Verification items for the finished model (mm, model axes). A direction names the side the tool comes from. Give positions to 0.01 mm unless a question says otherwise; leave off trailing zeros. Write each loop counter-clockwise with the first axis right and the second up, starting at its lowest first coordinate (ties: lowest second). Pieces come first, ordered by that corner, then holes. Notation, with made-up numbers: (31.25, 45) - (66.25, 45) arc R33 ccw to (66.25, 74) - close; hole circle Ø7 at (15, 8). An arc over 180 degrees is marked (long way). Answer as a JSON object with one key per item and string values. Group by question number.
Item 1: Go/stop test with a flat-tipped pin: pin 1 (9.5 mm diameter, centred on x = 59.82, y = 20.1, fed in from -Z). Record where the tip stops, or that it passes through.
Item 2: Draft check along Y on faces 3 (the face through (35, 39.933, 5)), 4 (the face through (36, 24.503, 5)), 5 (the face through (9.02, 14.24, 4.93)), 6 (the face through (0, 20, 5)). Enter one of: +Y half, -Y half, draft (parallel to the pull), parting line (faces both ways), or undercut.
Item 3: Sectioned sample at B-B, the plane y = 17.5. Record the boundary of the cut face in (x, z).
Item 4: Tool access check on faces 1 (the face through (36, 15.695, 5)), 2 (the face through (68.865, 22.222, 8.521)). Record the directions out of +Z, -Z, +X, -X, +Y, -Y that give a thin tool (end or side, any length) a straight path to the whole face; none if there is none.
Item 5: Sectioned sample at D-D, the plane x = 5. Record the boundary of the cut face in (y, z).
Item 6: Sectioned sample at C-C, the plane z = 2. Record the boundary of the cut face in (x, y), and give its area (3 significant figures).
Item 7: Sectioned sample at A-A, the plane x = 34. Record the boundary of the cut face in (y, z), and give its area (3 significant figures).
Item 8: Scan lines: line 1 along Y through (x, z) = (39, 1.5); line 2 along X through (y, z) = (22.5, 9.5); line 3 along X through (y, z) = (17.5, 1.5). Record each from-to range of solid material in increasing order. Write a range as [from, to].
```python
from build123d import *

# Parameters (mm, degrees)
SKETCH_W         = 70.38591
SKETCH_H         = 39.932888
SKETCH_R         = 6
PAD_DEPTH        = 10
CHAMFER_SIZE     = 3
CHAMFER001_SIZE2 = 5
CHAMFER001_SIZE  = 2


with BuildPart() as part:
    # Sketch → Pad (new body)
    with BuildSketch(Plane.XY):
        with Locations((35.192955, 19.966444)):
            Rectangle(SKETCH_W, SKETCH_H)
        with Locations((10.318798, 20.099125)):
            Circle(SKETCH_R, mode=Mode.SUBTRACT)
        with Locations((59.81543, 20.099125)):
            Circle(SKETCH_R, mode=Mode.SUBTRACT)
        with BuildLine():
            ThreePointArc((27.097306, 24.503486), (22.692945, 20.099125), (27.097306, 15.694764))
            Line((27.097306, 15.694764), (44.71476, 15.694764))
            ThreePointArc((44.71476, 15.694764), (49.119121, 20.099125), (44.71476, 24.503486))
            Line((44.71476, 24.503486), (27.097306, 24.503486))
        make_face(mode=Mode.SUBTRACT)
    extrude(amount=PAD_DEPTH)

    # Chamfer
    chamfer_edges = [part.edges().sort_by_distance(p)[0] for p in [
        (70.38591, 19.966444, 10),
    ]]
    chamfer(chamfer_edges, length=CHAMFER_SIZE)

    # Chamfer001
    chamfer001_edges = [part.edges().sort_by_distance(p)[0] for p in [
        (68.88591, 0, 8.5),
    ]]
    chamfer001_side = part.faces().sort_by_distance((34.972942, 0, 4.974262))[0]
    chamfer(chamfer001_edges, length=CHAMFER001_SIZE, length2=CHAMFER001_SIZE2, reference=chamfer001_side)


solid = part.part
```
Geometry check:
{
 "1": {"pin 1": "through"},
 "2": {"face 3": "+Y half", "face 4": "undercut", "face 5": "undercut", "face 6": "draft"},
 "3": {"outline": "(0, 0) - (4.91, 0) - (4.91, 10) - (0, 10) - close; (15.73, 0) - (23.54, 0) - (23.54, 10) - (15.73, 10) - close; (48.27, 0) - (54.41, 0) - (54.41, 10) - (48.27, 10) - close; (65.22, 0) - (70.39, 0) - (70.39, 7) - (67.39, 10) - (65.22, 10) - close"},
 "4": {"face 1": "+Z, -Z", "face 2": "+Z, +X, +Y, -Y"},
 "5": {"outline": "(0, 0) - (17.32, 0) - (17.32, 10) - (0, 10) - close; (22.88, 0) - (39.93, 0) - (39.93, 10) - (22.88, 10) - close"},
 "6": {"outline": "(0, 0) - (70.39, 0) - (70.39, 39.93) - (0, 39.93) - close; hole circle Ø12 at (10.32, 20.1); hole (27.1, 15.69) - (44.71, 15.69) arc R4.4 ccw to (44.71, 24.5) - (27.1, 24.5) arc R4.4 ccw to start; hole circle Ø12 at (59.82, 20.1)", "area": "2,370 mm^2"},
 "7": {"outline": "(0, 0) - (15.69, 0) - (15.69, 10) - (0, 10) - close; (24.5, 0) - (39.93, 0) - (39.93, 10) - (24.5, 10) - close", "area": "311 mm^2"},
 "8": {"line 1": "[0, 15.69], [24.5, 39.93]", "line 2": "[0, 4.82], [15.82, 23.4], [48.41, 54.32], [65.31, 67.89]", "line 3": "[0, 4.91], [15.73, 23.54], [48.27, 54.41], [65.22, 70.39]"}
}
